Build history of the part. All positions in model axes, mm. A direction names the side the tool comes from. Give positions to 0.01 mm unless a question says otherwise; leave off trailing zeros. Order: outer loops, then holes, each group sorted by start corner. A loop starts at its lowest first (then second) coordinate and runs counter-clockwise, first axis right, second up. Notation, with made-up numbers: (72, -3) - (81, -3) arc R30 cw to (81, 25) - close; hole circle Ø2 at (65.25, 31.25). An arc over 180 degrees is marked (long way). Use a Markdown table: item, result. Add a question column.
(1) Slice it at A-A (x = 0). Write the cut outline in (y, z).
(2) Flat gauge pins, fed straight in: pin 1 (7.5 mm diameter, centred on x = -0.5, y = 22.5, fed in from +Z); pin 2 (3.5 mm diameter, centred on x = 22, y = 17, fed in from +Z); pin 3 (2.5 mm diameter, centred on x = 23.5, z = -18.5, fed in from +Y); pin 4 (6 mm diameter, centred on x = 18, z = -6.5, fed in from -Y). Where does each tip first touch, or does it go through?
(3) Slice it at D-D (y = 24.5). Write the cut outline in (x, z).
(4) Mould opens along X. For faces 1 (the face through (-27, 17, -18)), 2 (the face through (3, 3, -5)), 3 (the face through (13, 15, -13)) say: +X half, -X half, draft (parallel to the pull), parting line (faces both ways), or undercut.
(5) Which spindle directions (+Z, -Z, +X, -X, +Y, -Y) get a long thin tool onto all of the face, cutting with end or side? Do faces 4 (the face through (-11.791, 25.93, -17.345)), 5 (the face through (-13, 15, -13)), 6 (the face through (10.5, 15, -11)). Say none if no direction does.
(6) Slice it at B-B (z = 3.5). Write the cut outline in (x, y), then the cut area to 3 significant figures.
(7) Slice it at C-C (y = 17). Count the separate pieces of the cut face and the enclosed holes in it, then the cut area to 3 significant figures.
(8) Wall check: line 1 (X direction, y = 23.5, z = -16.5); line 2 (Y direction, x = 22, z = -18.5); line 3 (X direction, y = 25.5, z = -10). Give the ranges that are in metal, low to high.
from build123d import *

# Parameters (mm, degrees)
BOX043_W               = 24
BOX043_H               = 42
BOX043_DEPTH           = 13
SKETCH021_R            = 5
EXTRUDE021_DEPTH       = 3
CYLINDER038_R          = 1.6
CYLINDER038_DEPTH      = 10
BOX042_W               = 12
BOX042_H               = 10
BOX042_DEPTH           = 5
CUT030_PLACEMENT_ANGLE = 180
CYLINDER037_R          = 1.6
CYLINDER037_DEPTH      = 10
BOX041_W               = 12
BOX041_H               = 10
BOX041_DEPTH           = 5
BOX040_W               = 3
BOX040_H               = 2
BOX040_DEPTH           = 2
CYLINDER036_R          = 1.25
CYLINDER036_DEPTH      = 10
CYLINDER035_R          = 1.25
CYLINDER035_DEPTH      = 10
EXTRUDE020_DEPTH       = 28


with BuildPart() as cube025:
    # Box043 → Box043 (new body)
    with BuildSketch(Plane(origin=(-12, -2, 12), x_dir=(1, 0, 0), z_dir=(0, 0, 1))):
        with Locations((12, 21)):
            Rectangle(BOX043_W, BOX043_H)
    extrude(amount=BOX043_DEPTH)


with BuildPart() as front_cover:
    # Sketch021 → Extrude021 (new body)
    with BuildSketch(Plane.XZ):
        with BuildLine():
            ThreePointArc((10, 11), (0, 22.517745), (-10, 11))
            ThreePointArc((-10, 11), (-15.587711, 0.627088), (-10.5, -10))
            Line((-10.5, -10), (-10.5, -13))
            Line((-10.5, -13), (-15, -13))
            Line((-15, -13), (-15, -20))
            Line((-15, -20), (15, -20))
            Line((15, -13), (15, -20))
            Line((10.5, -13), (15, -13))
            Line((10.5, -10), (10.5, -13))
            ThreePointArc((10.5, -10), (15.587711, 0.627088), (10, 11))
        make_face()
        Circle(SKETCH021_R, mode=Mode.SUBTRACT)
    extrude(amount=-EXTRUDE021_DEPTH)


with BuildPart() as cylinder038:
    # Cylinder038 → Cylinder038 (new body)
    with BuildSketch(Plane(origin=(22, 17, -22), x_dir=(1, 0, 0), z_dir=(0, 0, 1))):
        Circle(CYLINDER038_R)
    extrude(amount=CYLINDER038_DEPTH)


with BuildPart() as cut030:
    # Box042 → Box042 (new body)
    with BuildSketch(Plane(origin=(15, 12, -20), x_dir=(1, 0, 0), z_dir=(0, 0, 1))):
        with Locations((6, 5)):
            Rectangle(BOX042_W, BOX042_H)
    extrude(amount=BOX042_DEPTH)

    # Cut030: cut Cylinder038
    add(cylinder038.part, mode=Mode.SUBTRACT)


with BuildPart() as cut030_1:
    # Cut030 placement: moved
    add(cut030.part.moved(Location((0, 34, 0))).rotate(Axis((0, 34, 0), (0, 0, 1)), CUT030_PLACEMENT_ANGLE))


with BuildPart() as cylinder037:
    # Cylinder037 → Cylinder037 (new body)
    with BuildSketch(Plane(origin=(22, 17, -22), x_dir=(1, 0, 0), z_dir=(0, 0, 1))):
        Circle(CYLINDER037_R)
    extrude(amount=CYLINDER037_DEPTH)


with BuildPart() as cut029:
    # Box041 → Box041 (new body)
    with BuildSketch(Plane(origin=(15, 12, -20), x_dir=(1, 0, 0), z_dir=(0, 0, 1))):
        with Locations((6, 5)):
            Rectangle(BOX041_W, BOX041_H)
    extrude(amount=BOX041_DEPTH)

    # Cut029: cut Cylinder037
    add(cylinder037.part, mode=Mode.SUBTRACT)


with BuildPart() as cube022:
    # Box040 → Box040 (new body)
    with BuildSketch(Plane(origin=(-1.5, 29, 19.5), x_dir=(1, 0, 0), z_dir=(0, 0, 1))):
        with Locations((1.5, 1)):
            Rectangle(BOX040_W, BOX040_H)
    extrude(amount=BOX040_DEPTH)


with BuildPart() as cylinder036:
    # Cylinder036 → Cylinder036 (new body)
    with BuildSketch(Plane(origin=(-10.87, 21, -16.5), x_dir=(1, 0, 0), z_dir=(0, 1, 0))):
        Circle(CYLINDER036_R)
    extrude(amount=CYLINDER036_DEPTH)


with BuildPart() as m2_cyl:
    # Cylinder035 → Cylinder035 (new body)
    with BuildSketch(Plane(origin=(10.87, 21, -16.5), x_dir=(1, 0, 0), z_dir=(0, 1, 0))):
        Circle(CYLINDER035_R)
    extrude(amount=CYLINDER035_DEPTH)

    # Fusion024: union Cylinder036
    add(cylinder036.part)


with BuildPart() as outerbox:
    # Sketch020 → Extrude020 (new body)
    with BuildSketch(Plane.XZ):
        with BuildLine():
            ThreePointArc((10, 11), (0, 22.517745), (-10, 11))
            ThreePointArc((-10, 11), (-15.587711, 0.627088), (-10.5, -10))
            Line((-10.5, -10), (-10.5, -13))
            Line((-10.5, -13), (-15, -13))
            Line((-15, -13), (-15, -20))
            Line((-15, -20), (15, -20))
            Line((15, -13), (15, -20))
            Line((10.5, -13), (15, -13))
            Line((10.5, -10), (10.5, -13))
            ThreePointArc((10.5, -10), (15.587711, 0.627088), (10, 11))
        make_face()
        with BuildLine():
            Line((-7.5, -10), (-7.5, -16))
            Line((-7.5, -16), (7.5, -16))
            Line((7.5, -16), (7.5, -10))
            ThreePointArc((7.5, -10), (12.754076, 0.73948), (6.583703, 10.98))
            ThreePointArc((6.583703, 10.98), (0, 18.524934), (-6.583703, 10.98))
            ThreePointArc((-6.583703, 10.98), (-12.754076, 0.73948), (-7.5, -10))
        make_face(mode=Mode.SUBTRACT)
    extrude(amount=-EXTRUDE020_DEPTH)


with BuildPart() as outerbox_1:
    # Extrude020 placement: moved
    add(outerbox.part.moved(Location((0, 3, 0))))

    # Cut027: cut m2_cyl
    add(m2_cyl.part, mode=Mode.SUBTRACT)

    # Cut028: cut Cube022
    add(cube022.part, mode=Mode.SUBTRACT)

    # Fusion026: union Front_cover, Cut030, Cut029
    add(front_cover.part)
    add(cut030_1.part)
    add(cut029.part)

    # Cut031: cut Cube025
    add(cube025.part, mode=Mode.SUBTRACT)


solid = outerbox_1.part
Solution:
| question | item | result |
|---|---|---|
| 1 | outline | (0, -20) - (31, -20) - (31, -16) - (3, -16) - (3, -5) - (0, -5) - close; (0, 5) - (3, 5) - (3, 12) - (0, 12) - close |
| 2 | pin 1 | z = -16 |
| 2 | pin 2 | z = -15 |
| 2 | pin 3 | y = 22 |
| 2 | pin 4 | through |
| 3 | outline | (-15, -20) - (15, -20) - (15, -13) - (10.5, -13) - (10.5, -10) arc R13 ccw to (10, 11) arc R10.1 ccw to (10.09, 12) - (6.64, 12) arc R6.64 cw to (6.58, 10.98) arc R12.5 cw to (7.5, -10) - (7.5, -16) - (-7.5, -16) - (-7.5, -10) arc R12.5 cw to (-6.58, 10.98) arc R6.64 cw to (-6.64, 12) - (-10.09, 12) arc R10.1 ccw to (-10, 11) arc R13 ccw to (-10.5, -10) - (-10.5, -13) - (-15, -13) - close; hole circle Ø2.5 at (-10.87, -16.5); hole circle Ø2.5 at (10.87, -16.5) |
| 4 | face 1 | -X half |
| 4 | face 2 | undercut |
| 4 | face 3 | draft |
| 5 | face 4 | +Y |
| 5 | face 5 | -X, +Y, -Y |
| 5 | face 6 | +X, +Y, -Y |
| 6 | outline | (-15.2, 0) - (-3.57, 0) - (-3.57, 3) - (-12.32, 3) - (-12.32, 31) - (-15.2, 31) - close; (3.57, 0) - (15.2, 0) - (15.2, 31) - (12.32, 31) - (12.32, 3) - (3.57, 3) - close |
| 6 | area | 231 mm2 |
| 7 | separate pieces | 3 |
| 7 | enclosed holes | 0 |
| 7 | area | 400 mm2 |
| 8 | line 1 | -15 to -12.12, -9.62 to 9.62, 12.12 to 15 |
| 8 | line 2 | 12 to 15.4, 18.6 to 22 |
| 8 | line 3 | -10.5 to -7.5, 7.5 to 10.5 |
